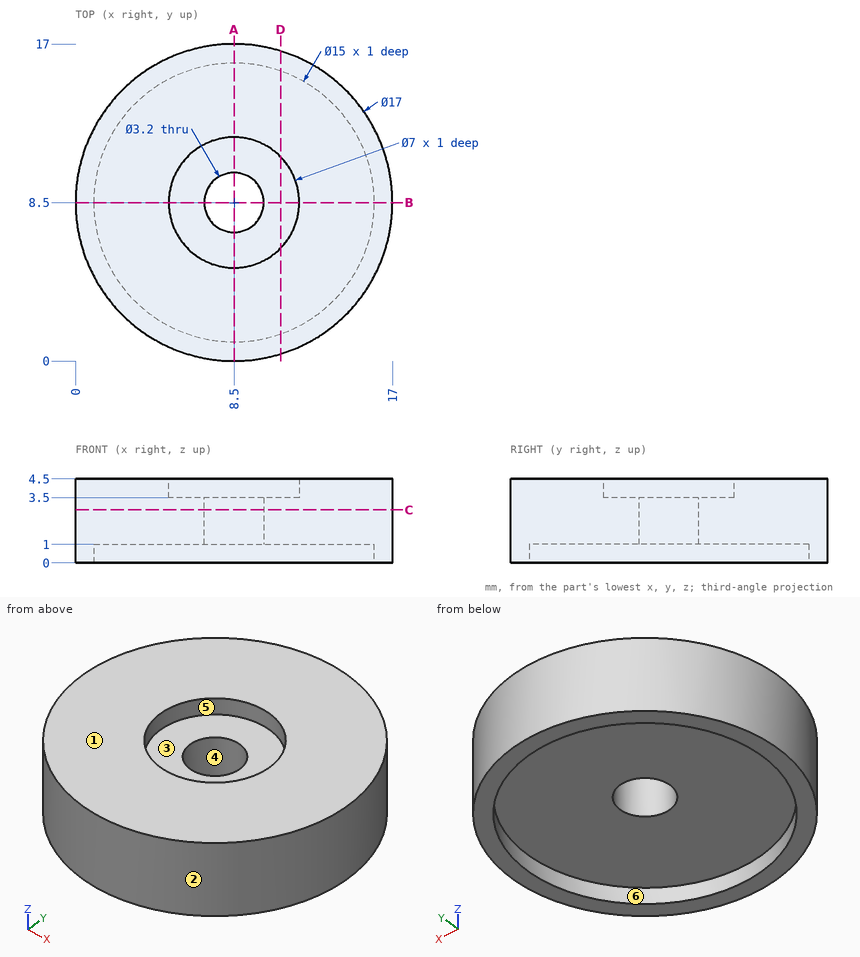
Input: dimensioned drawing with shaded views. Units: mm. Origin: part minimum x, y, z. A direction names the side the tool comes from. Coordinates: 2 decimals unless noted, no trailing zeros. Write each loop counter-clockwise with the first axis right and the second up, starting at its lowest first coordinate (ties: lowest second). Pieces come first, ordered by that corner, then holes. Notation, with made-up numbers: (-26, 60) -> (8, 60) arc R25 cw to (8, 96) -> close; hole circle Ø8 at (-15, 20). An arc over 180 degrees is marked (long way). Return JSON: item names as keys, results as strings. Group by question number.
1) Ray query, line 1 along Y through (x, z) = (8.5, 4); line 2 along Y through (x, z) = (8.5, 0.6); line 3 along X through (y, z) = (8.25, 3.6). Return the intervals inside material, ascending.
2) Section query D-D, the plane x = 11. Return loops of the section in (y, z), plus the area to 3 significant figures.
3) Section query C-C, the plane z = 2.85. Return loops of the section in (x, y), plus the area to 3 significant figures.
4) Contact query for flat-ended pins moving along their axis: P1, Ø2, axis at x = 12, z = 0.5, coming from the +Y side; P2, Ø6.5, axis at x = 8.5, y = 8.5, coming from the -Z side; P3, Ø3.5, axis at x = 8.5, y = 8.5, coming from the +Z side. Output: stop coordinate, or through.
5) Set-up query: the marked faces 4, 5 and 6. Return all of +Z, -Z, +X, -X, +Y, -Y with unobstructed straight access to the full face (end or side cutting, diameter ignored); none if empty.
6) Section query A-A, the plane x = 8.5. Return loops of the section in (y, z).
7) Mould query, pull axis Y, two halves, no side actions, for the marked faces 1, 2 and 3. Classes: +Y half, -Y half, draft (parallel to the pull), parting line (faces both ways), or undercut.
From the geometry:
{
 "1": {"line 1": "0 to 5, 12 to 17", "line 2": "0 to 1, 16 to 17", "line 3": "0 to 5.01, 11.99 to 17"},
 "2": {"outline": "(0.38, 0) -> (1.43, 0) -> (1.43, 1) -> (15.57, 1) -> (15.57, 0) -> (16.62, 0) -> (16.62, 4.5) -> (10.95, 4.5) -> (10.95, 3.5) -> (6.05, 3.5) -> (6.05, 4.5) -> (0.38, 4.5) -> close", "area": "54.1 mm²"},
 "3": {"outline": "circle Ø17 at (8.5, 8.5); hole circle Ø3.2 at (8.5, 8.5)", "area": "219 mm²"},
 "4": {"P1": "y = 16.62", "P2": "z = 1", "P3": "z = 3.5"},
 "5": {"face 4": "+Z, -Z", "face 5": "+Z", "face 6": "-Z"},
 "6": {"outline": "(0, 0) -> (1, 0) -> (1, 1) -> (6.9, 1) -> (6.9, 3.5) -> (5, 3.5) -> (5, 4.5) -> (0, 4.5) -> close; (10.1, 1) -> (16, 1) -> (16, 0) -> (17, 0) -> (17, 4.5) -> (12, 4.5) -> (12, 3.5) -> (10.1, 3.5) -> close"},
 "7": {"face 1": "draft", "face 2": "parting line", "face 3": "undercut"}
}
